Part model, mm, in its own coordinate system. A direction names the side the tool comes from. Give positions to 0.01 mm unless a question says otherwise; leave off trailing zeros. Write each loop counter-clockwise with the first axis right and the second up, starting at its lowest first coordinate (ties: lowest second). Pieces come first, ordered by that corner, then holes.
```python
from build123d import *

# Parameters (mm, degrees)
F0_W     = 3.1029209495
F0_H     = 8
F0_R     = 1.25
F1_DEPTH = 7
F0_R_2   = 1.75
F2_DEPTH = 12
F0_W_2   = 30
F0_H_2   = 40
F3_DEPTH = 7
F4_R     = 5
F5_R     = 1.75
F6_DEPTH = 25
F0_W_3   = 50
F0_H_3   = 15
F7_DEPTH = 4


with BuildPart() as f1:
    # F0 (on Top) → F1 (new body)
    with BuildSketch(Plane.XY):
        Polygon((25, -50), (25, 65), (-25, 65), (-25, -5), (-25, -45), (-25, -50), align=None)
        with Locations((-20.4485395253, -41)):
            Rectangle(F0_W, F0_H, mode=Mode.SUBTRACT)
        with Locations((20.4485395253, -41)):
            Rectangle(F0_W, F0_H, mode=Mode.SUBTRACT)
        with Locations((-20.4485395253, 12)):
            Rectangle(F0_W, F0_H, mode=Mode.SUBTRACT)
        with Locations((-18.25, 33.75)):
            Circle(F0_R, mode=Mode.SUBTRACT)
        with Locations((20.4485395253, 12)):
            Rectangle(F0_W, F0_H, mode=Mode.SUBTRACT)
        Polygon((15.25, 40), (15.25, 27.5), (-15.25, 27.5), (-15.25, 31.75), (-16.25, 31.75), (-16.25, 35.75), (-15.25, 35.75), (-15.25, 40), align=None, mode=Mode.SUBTRACT)
        with Locations((18.25, 33.75)):
            Circle(F0_R, mode=Mode.SUBTRACT)
    extrude(amount=F1_DEPTH)

    # F0 (on Top) → F2 (join)
    with BuildSketch(Plane.XY):
        with BuildLine():
            Line((-25, 65), (25, 65))
            Line((25, 65), (45, 65))
            ThreePointArc((45, 65), (48.5355339059, 66.4644660941), (50, 70))
            ThreePointArc((50, 70), (48.5355339059, 73.5355339059), (45, 75))
            Line((45, 75), (-45, 75))
            ThreePointArc((-45, 75), (-48.5355339059, 73.5355339059), (-50, 70))
            ThreePointArc((-50, 70), (-48.5355339059, 66.4644660941), (-45, 65))
            Line((-45, 65), (-25, 65))
        make_face()
        with Locations((-44.2887660861, 70)):
            Circle(F0_R_2, mode=Mode.SUBTRACT)
        with Locations((45, 70)):
            Circle(F0_R_2, mode=Mode.SUBTRACT)
    extrude(amount=F2_DEPTH)

    # F0 (on Top) → F3 (join)
    with BuildSketch(Plane.XY):
        with Locations((-40, -25)):
            Rectangle(F0_W_2, F0_H_2)
    extrude(amount=F3_DEPTH)

    # F4
    f4_edges = [f1.edges().sort_by_distance(p)[0] for p in [
        (-55, -5, 3.5),
        (-55, -45, 3.5),
    ]]
    fillet(f4_edges, radius=F4_R)

    # F5 (on face) → F6 (cut)
    with BuildSketch(Plane.XY.offset(7)):
        with Locations((-50, -10)):
            Circle(F5_R)
        with Locations((-30, -10)):
            Circle(F5_R)
        with Locations((-30, -40)):
            Circle(F5_R)
        with Locations((-50, -40)):
            Circle(F5_R)
    extrude(amount=-F6_DEPTH, mode=Mode.SUBTRACT)

    # F0 (on Top) → F7 (join)
    with BuildSketch(Plane.XY):
        with Locations((0, -57.5)):
            Rectangle(F0_W_3, F0_H_3)
    extrude(amount=F7_DEPTH)


solid = f1.part
```
1) Saw through at A-A, the plane x = -6. Write the cut outline in (y, z), then the cut area to 4 significant figures.
Answers follow:
outline: (-65, 0) - (27.5, 0) - (27.5, 7) - (-50, 7) - (-50, 4) - (-65, 4) - close; (40, 0) - (75, 0) - (75, 12) - (65, 12) - (65, 7) - (40, 7) - close
area: 897.5 mm2
2) 3-axis set-ups, long thin cutter, end or side, ignore diameter. For faces 4 (the face through (0, -57, 4)), 5 (the face through (22, -41, 3)), 6 (the face through (-38, -5, 3)), 7 (the face through (-55, -25, 3)), 8 (the face through (-54, -43, 4)): which of +Z, -Z, +X, -X, +Y, -Y reach the whole face in a straight line?
Answers follow:
face 4: +Z, +X, -X, -Y
face 5: +Z, -Z
face 6: +Z, -Z, -X
face 7: +Z, -Z, -X, +Y, -Y
face 8: +Z, -Z, -X, -Y
3) Saw through at B-B, the plane x = -30. Write the cut outline in (y, z), then the cut area to 3 significant figures.
Answers follow:
outline: (-45, 0) - (-41.75, 0) - (-41.75, 7) - (-45, 7) - close; (-38.25, 0) - (-11.75, 0) - (-11.75, 7) - (-38.25, 7) - close; (-8.25, 0) - (-5, 0) - (-5, 7) - (-8.25, 7) - close; (65, 0) - (75, 0) - (75, 12) - (65, 12) - close
area: 351 mm2
4) Two-plate mould, pull along Y, no slides. Class faces 1 (the face through (1, 75, 6)), 2 (the face through (0, -65, 2)), 3 (the face through (18.897, 12, 3)): +Y half, -Y half, draft (parallel to the pull), parting line (faces both ways), or undercut.
Answers follow:
face 1: +Y half
face 2: -Y half
face 3: undercut
5) Saw through at D-D, the plane z = 1.75. Count the separate pieces of the cut face and the enclosed holes in it, then the cut area to 3 significant figures.
Answers follow:
separate pieces: 1
enclosed holes: 13
area: 8,120 mm2
6) Pin check, flat tips, straight feed: pin 1 Ø6 at (x, y) = (-32, -21.5) entering from +Z; pin 2 Ø3 at (y, z) = (34.5, 4.5) entering from +X; pin 3 Ø10 at (x, y) = (-12.5, 6.5) entering from -Z; pin 4 Ø6 at (x, z) = (-4, 9) entering from -Y. Stop position of each tip, or through.
Answers follow:
pin 1: stops at z = 7
pin 2: stops at x = 25
pin 3: stops at z = 0
pin 4: stops at y = -50
7) Saw through at C-C, the plane z = 9.25. Write the cut outline in (x, y).
Answers follow:
outline: (-45, 65) - (45, 65) arc R5 ccw to (45, 75) - (-45, 75) arc R5 ccw to start; hole circle Ø3.5 at (-44.29, 70); hole circle Ø3.5 at (45, 70)
8) Wall check: L1, parallel to Y at x = -30, z = 5.25; L2, parallel to Y at x = 8, z = 2.25; L3, parallel to Y at x = -18.25, z = 5.75. Give the ranges that are in metal, low to high.
Answers follow:
L1: y = -45 to -41.75, -38.25 to -11.75, -8.25 to -5, 65 to 75
L2: y = -65 to 27.5, 40 to 75
L3: y = -50 to 32.5, 35 to 75
